Check sheet for the modelled part. Datum: model origin and axes. Units: mm. Face numbers are marked on the shaded views. A direction names the side the tool comes from. Round coordinates to 2 decimals unless told otherwise and drop trailing zeros. Write each loop counter-clockwise with the first axis right and the second up, starting at its lowest first coordinate (ties: lowest second). Pieces come first, ordered by that corner, then holes. Notation, with made-up numbers: M -18,8 L 5,8 A26 cw 5,33 Z; hole C 40.5,30 d4. An arc over 180 degrees is marked long. One line per item, written item: value.
from build123d import *

# Parameters (mm, degrees)
SKETCH1_W           = 12.7
SKETCH1_H           = 23.7
BOSS_EXTRUDE1_DEPTH = 2
SKETCH2_W           = 12.7
SKETCH2_H           = 17
BOSS_EXTRUDE2_DEPTH = 2
SKETCH3_W           = 12.7
SKETCH3_H           = 17
BOSS_EXTRUDE3_DEPTH = 2
SKETCH4_W           = 27.7
SKETCH4_H           = 17
BOSS_EXTRUDE4_DEPTH = 2
SKETCH5_W           = 27.7
SKETCH5_H           = 17
BOSS_EXTRUDE5_DEPTH = 2
CUT_EXTRUDE2_REACH  = 36.141
SKETCH7_W           = 5
SKETCH7_H           = 12.5


with BuildPart() as part:
    # Sketch1 → Boss-Extrude1 (new body)
    with BuildSketch(Plane(origin=(0, 0, 0), x_dir=(1, 0, 0), z_dir=(0, 1, 0))):
        with Locations((6.35, 11.85)):
            Rectangle(SKETCH1_W, SKETCH1_H)
    extrude(amount=BOSS_EXTRUDE1_DEPTH)

    # Sketch2 → Boss-Extrude2 (add)
    with BuildSketch(Plane.XY):
        with Locations((6.35, 8.5)):
            Rectangle(SKETCH2_W, SKETCH2_H)
    extrude(amount=BOSS_EXTRUDE2_DEPTH)

    # Sketch3 → Boss-Extrude3 (add)
    with BuildSketch(Plane(origin=(0, 0, -23.7), x_dir=(-1, 0, 0), z_dir=(0, 0, -1))):
        with Locations((-6.35, 8.5)):
            Rectangle(SKETCH3_W, SKETCH3_H)
    extrude(amount=BOSS_EXTRUDE3_DEPTH)

    # Sketch4 → Boss-Extrude4 (add)
    with BuildSketch(Plane(origin=(12.7, 0, 0), x_dir=(0, 0, -1), z_dir=(1, 0, 0))):
        with Locations((11.85, 8.5)):
            Rectangle(SKETCH4_W, SKETCH4_H)
    extrude(amount=BOSS_EXTRUDE4_DEPTH)

    # Sketch5 → Boss-Extrude5 (add)
    with BuildSketch(Plane.ZY):
        with Locations((-11.85, 8.5)):
            Rectangle(SKETCH5_W, SKETCH5_H)
    extrude(amount=BOSS_EXTRUDE5_DEPTH)

    # Sketch7 → Cut-Extrude2 (cut, up to next)
    with BuildSketch(Plane.XY.offset(-23.7), mode=Mode.PRIVATE) as cut_extrude2_sk1:
        with Locations((6.35, 10.75)):
            Rectangle(SKETCH7_W, SKETCH7_H)
    cut_extrude2_tool1 = extrude(cut_extrude2_sk1.sketch, amount=-CUT_EXTRUDE2_REACH, mode=Mode.PRIVATE) & part.part
    add(cut_extrude2_tool1.solids().sort_by_distance((6.35, 10.75, -23.7))[0], mode=Mode.SUBTRACT)


solid = part.part
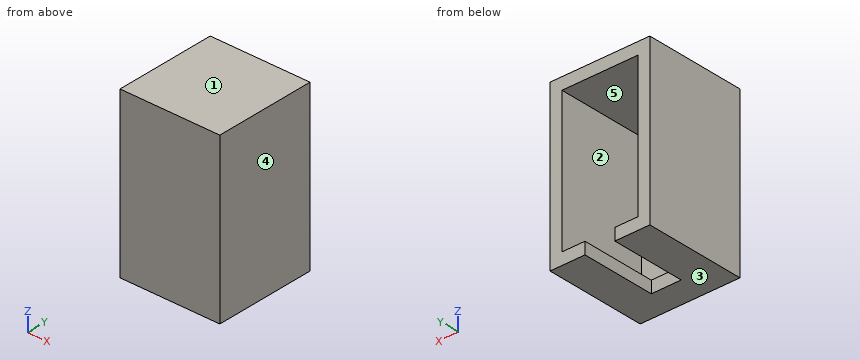
Q1. Depth check by flat-ended pin: P1, Ø2, axis at x = 5.5, z = -24.5, coming from the +Y side; P2, Ø4, axis at x = 9, z = -12, coming from the +Y side; P3, Ø2, axis at x = 6.5, z = -11, coming from the -Y side. Enter the tip coordinate at first touch or a pass-through.
Completed:
P1: y = 4.5
P2: y = 2
P3: y = 0
Q2. Sectioned sample at A-A on y = 15.5. Enter the section's corners in (x, z), and give its area (3 significant figures).
Completed:
outline: M -2,-25.7 L 3.85,-25.7 L 3.85,-23.7 L 0,-23.7 L 0,0 L 12.7,0 L 12.7,-23.7 L 8.85,-23.7 L 8.85,-25.7 L 14.7,-25.7 L 14.7,2 L -2,2 Z
area: 152 mm^2
Q3. Sectioned sample at B-B on x = 10.25. Enter the section's corners in (y, z).
Completed:
outline: M 0,-25.7 L 17,-25.7 L 17,-23.7 L 2,-23.7 L 2,0 L 17,0 L 17,2 L 0,2 Z
Q4. Draft check along X on the marked faces 3, 4 and 5. Enter one of: pulls with the +X half, pulls with the -X half, needs draft (parallel to the pull), parting line crosses it, or undercut.
Completed:
face 3: needs draft
face 4: pulls with the +X half
face 5: undercut
Q5. Scan lines: line 1 (Z direction, x = 3.75, y = 10.25); line 2 (X direction, y = 14.5, z = -7.25); line 3 (Z direction, x = 5, y = 9.5). Record each from-to range of solid material in increasing order. Write a range as [from, to].
Completed:
line 1: [-25.7, -23.7], [0, 2]
line 2: [-2, 0], [12.7, 14.7]
line 3: [0, 2]
Q6. Access from +Z, -Z, +X, -X, +Y, -Y to the whole of each face (thin tool, end or side, straight path). Record for the marked faces 1 and 2.
Completed:
face 1: +Z, +X, -X, +Y, -Y
face 2: +Y
Q7. Sectioned sample at C-C on z = -15.25. Enter the section's corners in (x, y), and give its area (3 significant figures).
Completed:
outline: M -2,0 L 14.7,0 L 14.7,17 L 12.7,17 L 12.7,2 L 0,2 L 0,17 L -2,17 Z
area: 93.4 mm^2
